Here's how the part is built. I have some questions about the finished solid (model axes, mm). A direction names the side the tool comes from. Round coordinates to 2 decimals unless told otherwise and drop trailing zeros. Order: outer loops, then holes, each group sorted by start corner. A loop starts at its lowest first (then second) coordinate and runs counter-clockwise, first axis right, second up. Notation, with made-up numbers: (55, 64) - (90, 64) arc R18 ccw to (90, 82) - close; hole circle Ø1 at (71, 6.5). An arc over 180 degrees is marked (long way). One line per item, written item: value.
from build123d import *

# Parameters (mm, degrees)
SKETCH12_W                = 35
SKETCH12_H                = 44
CHAMBER_DEPTH             = 16
SKETCH13_R                = 11.5
BODY_DEPTH                = 31
HOT_END_TONEL_DEPTH       = 76.538069872
SKETCH26_W                = 27
SKETCH26_H                = 1.5
GRID_V_DEPTH              = 6
GRID_H_DEPTH              = 16
SKETCH16_R                = 13.5
SKETCH18_R                = 11.5
SKETCH20_R                = 8.125
HOT_END_1_DEPTH           = 3.2
SKETCH21_R                = 7
HOT_END_2_DEPTH           = 5.6
SKETCH22_R                = 8.125
HOT_END_3_DEPTH           = 4.2
SKETCH24_R                = 1.825
MOUNT_HOLES_DEPTH         = 71.156967099
SKETCH25_R                = 1.75
FAN_MOUNT_HOLES_DEPTH     = 8
FAN_MOUNT_NUT_HOLES_START = -2
FAN_MOUNT_NUT_HOLES_DEPTH = 2.6
SKETCH32_R                = 1.825
HOT_END_SCREW_HOLE_DEPTH  = 20
HOT_END_NUT_HOLE_START    = 2.5
HOT_END_NUT_HOLE_DEPTH    = 2.6
SKETCH35_R                = 1.825
BOSS_EXTRUDE1_DEPTH       = 5
CUT_EXTRUDE5_DEPTH        = 3
SKETCH37_R                = 3.6
CUT_EXTRUDE6_DEPTH        = 3
FILLET1_R                 = 3


with BuildPart() as part:
    # Sketch12 → chamber (new body)
    with BuildSketch(Plane(origin=(0, 0, 0), x_dir=(-1, 0, 0), z_dir=(0, -1, 0))):
        with Locations((3.5, -43)):
            Rectangle(SKETCH12_W, SKETCH12_H)
    extrude(amount=-CHAMBER_DEPTH)

    # Sketch13 → body (cut)
    with BuildSketch(Plane.XY.offset(65)):
        with Locations((-3.5, 16)):
            Circle(SKETCH13_R)
    extrude(amount=-BODY_DEPTH, mode=Mode.SUBTRACT)

    # Sketch14 → hot-end-tonel (cut, through all)
    with BuildSketch(Plane(origin=(14, 0, 0), x_dir=(0, 0, -1), z_dir=(1, 0, 0))):
        with BuildLine():
            Line((-51, 27.5), (-47, 27.5))
            ThreePointArc((-47, 27.5), (-35.5, 16), (-47, 4.5))
            Line((-47, 4.5), (-51, 4.5))
            ThreePointArc((-51, 4.5), (-62.5, 16), (-51, 27.5))
        make_face()
    extrude(amount=-HOT_END_TONEL_DEPTH, mode=Mode.SUBTRACT)

    # Sketch26 → grid-v (add)
    with BuildSketch(Plane(origin=(14, 0, 0), x_dir=(0, 0, -1), z_dir=(1, 0, 0))):
        with Locations((-49, 11.25)):
            Rectangle(SKETCH26_W, SKETCH26_H)
    extrude(amount=-GRID_V_DEPTH)

    # Sketch27 → grid-h (add)
    with BuildSketch(Plane.XZ):
        Polygon((8, 56), (14, 53), (14, 52), (8, 55), align=None)
        Polygon((14, 44), (8, 47), (8, 48), (14, 45), align=None)
    extrude(amount=-GRID_H_DEPTH)

    # Sketch16 → Cut-Loft1 section 0
    with BuildSketch(Plane(origin=(-21, 0, 0), x_dir=(0, 0, -1), z_dir=(1, 0, 0))):
        with Locations((-49, 16)):
            Circle(SKETCH16_R)
    # Sketch18 → Cut-Loft1 section 1
    with BuildSketch(Plane.ZY.offset(17)):
        with Locations((49, 16)):
            Circle(SKETCH18_R)
    loft(mode=Mode.SUBTRACT)

    # Sketch20 → hot-end-1 (cut)
    with BuildSketch(Plane.XY.offset(34)):
        with Locations((-3.5, 16)):
            Circle(SKETCH20_R)
    extrude(amount=-HOT_END_1_DEPTH, mode=Mode.SUBTRACT)

    # Sketch21 → hot-end-2 (cut)
    with BuildSketch(Plane.XY.offset(30.8)):
        with Locations((-3.5, 16)):
            Circle(SKETCH21_R)
    extrude(amount=-HOT_END_2_DEPTH, mode=Mode.SUBTRACT)

    # Sketch22 → hot-end-3 (cut)
    with BuildSketch(Plane.XY.offset(25.2)):
        with Locations((-3.5, 16)):
            Circle(SKETCH22_R)
    extrude(amount=-HOT_END_3_DEPTH, mode=Mode.SUBTRACT)

    # Sketch24 → mount-holes (cut, through all)
    with BuildSketch(Plane.XZ):
        with Locations(Location((-15.5, 28, 0), (0, 0, 270))):
            Circle(SKETCH24_R)
        with Locations(Location((8.5, 28, 0), (0, 0, 270))):
            Circle(SKETCH24_R)
    extrude(amount=-MOUNT_HOLES_DEPTH, mode=Mode.SUBTRACT)

    # Sketch25 → fan-mount-holes (cut)
    with BuildSketch(Plane.ZY.offset(21)):
        with Locations((60.999999795, 4)):
            Circle(SKETCH25_R)
        with Locations((36.999999795, 4)):
            Circle(SKETCH25_R)
    extrude(amount=-FAN_MOUNT_HOLES_DEPTH, mode=Mode.SUBTRACT)

    # Sketch34 → fan-mount-nut-holes (cut)
    with BuildSketch(Plane.ZY.offset(21).offset(FAN_MOUNT_NUT_HOLES_START)):
        Polygon((33.949999795, 0), (40.049999795, 0), (40.049999795, 5.760918321), (36.999999795, 7.521836642), (33.949999795, 5.760918321), align=None)
        Polygon((64.049999795, 0), (64.049999795, 5.760918321), (60.999999795, 7.521836642), (57.949999795, 5.760918321), (57.949999795, 0), align=None)
    extrude(amount=-FAN_MOUNT_NUT_HOLES_DEPTH, mode=Mode.SUBTRACT)


with BuildPart() as body_2:
    # Mirror1: mirrored copy
    add(part.part.mirror(Plane.ZX.offset(16)))

    # Sketch32 → hot-end-screw-hole (cut)
    with BuildSketch(Plane(origin=(0, 32, 0), x_dir=(-1, 0, 0), z_dir=(0, -1, 0))):
        with Locations(Location((3.5, -28, 0), (0, 0, 270))):
            Circle(SKETCH32_R)
    extrude(amount=HOT_END_SCREW_HOLE_DEPTH, mode=Mode.SUBTRACT)

    # Sketch33 → hot-end-nut-hole (cut)
    with BuildSketch(Plane.XZ.offset(-32).offset(HOT_END_NUT_HOLE_START)):
        Polygon((-6.55, 21), (-0.45, 21), (-0.45, 29.760918321), (-3.5, 31.521836642), (-6.55, 29.760918321), align=None)
    extrude(amount=HOT_END_NUT_HOLE_DEPTH, mode=Mode.SUBTRACT)

    # Sketch35 → Boss-Extrude1 (add)
    # profile 1 of 2: a face of its own
    with BuildSketch(Plane(origin=(0, 32, 0), x_dir=(1, 0, 0), z_dir=(0, 1, 0))):
        with BuildLine():
            Line((9.305077899, -65), (14.504047822, -69.701151268))
            ThreePointArc((14.504047822, -69.701151268), (23.208629379, -72.853515786), (19.198969923, -64.509070137))
            Line((19.198969923, -64.509070137), (14, -59.807918869))
            Line((14, -59.807918869), (9.305077899, -65))
        make_face()
        with Locations(Location((19.5, -69.5, 0), (0, 0, 270))):
            Circle(SKETCH35_R, mode=Mode.SUBTRACT)
    # profile 2 of 2: a face of its own
    with BuildSketch(Plane(origin=(0, 32, 0), x_dir=(1, 0, 0), z_dir=(0, 1, 0))):
        with BuildLine():
            Line((14, -39.5), (14, -29.5))
            Line((14, -29.5), (19.5, -29.5))
            ThreePointArc((19.5, -29.5), (24.5, -34.5), (19.5, -39.5))
            Line((19.5, -39.5), (14, -39.5))
        make_face()
        with Locations(Location((19.5, -34.5, 0), (0, 0, 270))):
            Circle(SKETCH35_R, mode=Mode.SUBTRACT)
    extrude(amount=-BOSS_EXTRUDE1_DEPTH)

    # Sketch36 → Cut-Extrude5 (cut)
    with BuildSketch(Plane.XZ.offset(-27)):
        Polygon((17.739081679, 31.45), (21.260918321, 31.45), (23.021836642, 34.5), (21.260918321, 37.55), (17.739081679, 37.55), (15.978163358, 34.5), align=None)
        Polygon((23.021836642, 69.5), (21.260918321, 72.55), (17.739081679, 72.55), (15.978163358, 69.5), (17.739081679, 66.45), (21.260918321, 66.45), align=None)
    extrude(amount=-CUT_EXTRUDE5_DEPTH, mode=Mode.SUBTRACT)

    # Sketch37 → Cut-Extrude6 (cut)
    with BuildSketch(Plane(origin=(0, 32, 0), x_dir=(1, 0, 0), z_dir=(0, 1, 0))):
        with Locations(Location((-15.5, -28, 0), (0, 0, 270))):
            Circle(SKETCH37_R)
        with Locations(Location((8.5, -28, 0), (0, 0, 270))):
            Circle(SKETCH37_R)
    extrude(amount=-CUT_EXTRUDE6_DEPTH, mode=Mode.SUBTRACT)

    # Fillet1
    fillet1_edges = [body_2.edges().sort_by_distance(p)[0] for p in [
        (14, 29.5, 59.807918869),
        (14, 29.5, 29.5),
        (14, 29.5, 39.5),
    ]]
    fillet(fillet1_edges, radius=FILLET1_R)


solid = body_2.part
Q1. If we section it at A-A, the plane x = 18.5: Please give me the cut outline in (y, z), then the cut area to 3 significant figures.
Results list:
outline: (27, 29.5) - (32, 29.5) - (32, 32.97) - (30, 32.97) - (30, 31.45) - (27, 31.45) - close; (27, 37.55) - (30, 37.55) - (30, 36.03) - (32, 36.03) - (32, 39.5) - (27, 39.5) - close; (27, 63.88) - (32, 63.88) - (32, 67.97) - (30, 67.97) - (30, 66.45) - (27, 66.45) - close; (27, 72.55) - (30, 72.55) - (30, 71.03) - (32, 71.03) - (32, 74.4) - (27, 74.4) - close
area: 53.8 mm²
Q2. If we section it at B-B, the plane z = 60: Give the number of separate pieces and of enclosed holes in the cut face, then the cut area to 3 significant figures.
Results list:
separate pieces: 3
enclosed holes: 0
area: 232 mm²
Q3. We'd pull the mould along Y, two halves only. Please class faces 4 (the flat face through (-13, 28, 37)), 5 (the cylindrical face through (-14.7, 26.5, 37.9)), 6 (the flat face through (-15, 29, 26)), 7 (the cylindrical face through (-3.753, 27.497, 37.702)): released by +Y, released by -Y, zero draft, split by the parting line, or undercut.
Results list:
face 4: undercut
face 5: undercut
face 6: released by +Y
face 7: released by -Y
Q4. Will these pins go through, and if not, where does the flat tip stop? pin 1 (1.2 mm diameter, centred on x = 6, z = 49, fed in from -Y); pin 2 (5 mm diameter, centred on x = -7.5, y = 23.5, fed in from +Z); pin 3 (1.8 mm diameter, centred on y = 28.5, z = 37, fed in from -X).
Results list:
pin 1: y = 27.5
pin 2: z = 34
pin 3: x = -13
Q5. Which directions (+Z, -Z, +X, -X, +Y, -Y) give clear straight access to the entire face, cutting with the end or side of a thin tool? Please do faces 1 (the flat face through (22.154, 28.479, 71.004)), 2 (the cylindrical face through (-3.679, 24.123, 32.422)), 3 (the flat face through (-18, 29, 57.95)).
Results list:
face 1: -Y
face 2: +Z, -Y
face 3: +Y
Q6. If I drill on line 1 along Z through (x, y) = (-14.3, 28) (3 decimals); line 2 along Z through (x, y) = (-14.75, 28); line 3 along X through (y, z) = (29.25, 30.5), over which ranges is the centre line in solid material (lowest first)?
Results list:
line 1: 21 to 26.625, 29.375 to 35.25, 38.75 to 59.25, 62.75 to 65
line 2: 21 to 26.34, 29.66 to 35.25, 38.75 to 59.25, 62.75 to 65
line 3: -21 to -18.09, -12.91 to -5.27, -1.73 to 5.91, 11.09 to 22.5
